Study the drawing (mm; zero at the part's minimum x, y, z) and answer. A direction names the side the tool comes from. Give positions to 0.01 mm unless a question says otherwise; leave off trailing zeros. Order: outer loops, then holes, each group sorted by start corner. A loop starts at its lowest first (then second) coordinate and runs counter-clockwise, first axis right, second up.
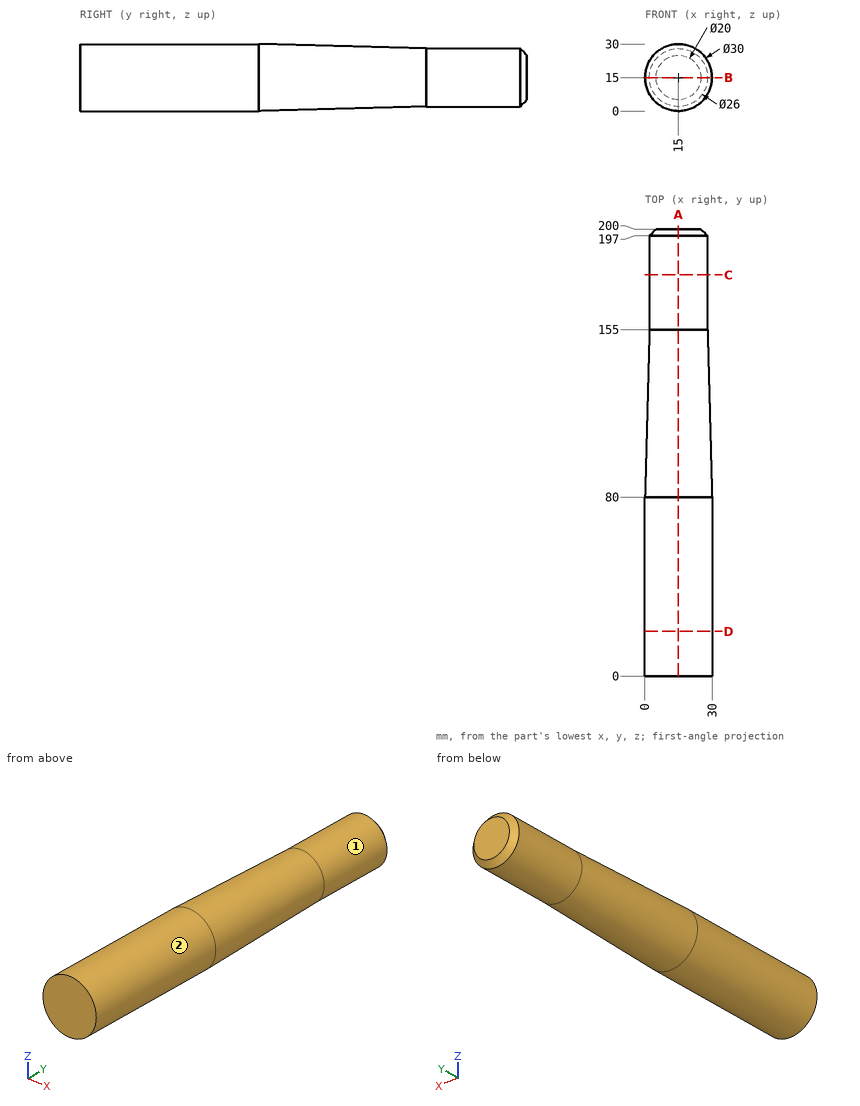
1) A tool of negligible diameter and unlimited length cuts with its end or side. For the marked faces 1 and 2, from which of +Z, -Z, +X, -X, +Y, -Y can it reach the whole face along a straight path? Write none if from no direction.
Geometry says:
face 1: +Y
face 2: +Y, -Y
2) Find section C-C (y = 179.5). Write down the section's boundary in (x, z), then the cut area to 3 significant figures.
Geometry says:
outline: circle Ø26 at (15, 15)
area: 531 mm2
3) Find section B-B (z = 15). Write down the section's boundary in (x, y), then the cut area to 3 significant figures.
Geometry says:
outline: (0, 0) - (30, 0) - (30, 80) - (28, 155) - (28, 197) - (25, 200) - (5, 200) - (2, 197) - (2, 155) - (0, 80) - close
area: 5,660 mm2
4) Straight lines are drawn through the part: probe 1 along Z at (x, y) = (26, 34); probe 2 along X at (y, z) = (33, 23.5); probe 3 along Y at (x, z) = (23, 24). For each, find the intervals that lie inside material, in ascending order.
Geometry says:
probe 1: z = 4.8 to 25.2
probe 2: x = 2.64 to 27.36
probe 3: y = 0 to 197.96
5) Find section D-D (y = 20). Write down the section's boundary in (x, z).
Geometry says:
outline: circle Ø30 at (15, 15)
6) Given P1, Ø10, axis at x = 3.5, y = 160, coming from the -Z side; P2, Ø8, axis at y = 97, z = 17.5, coming from the +X side; P3, Ø4, axis at x = 25.5, y = 95.5, coming from the +Z side, each flat-ended and moving along its own axis, determine where each tip first touches the part or whether it passes through.
Geometry says:
P1: stops at z = 3.74
P2: stops at x = 29.63
P3: stops at z = 26.86
7) Find section A-A (x = 15). Write down the section's boundary in (y, z), then the cut area to 3 significant figures.
Geometry says:
outline: (0, 0) - (80, 0) - (155, 2) - (197, 2) - (200, 5) - (200, 25) - (197, 28) - (155, 28) - (80, 30) - (0, 30) - close
area: 5,660 mm2
